Input: dimensioned drawing with shaded views. Units: mm. Origin: part minimum x, y, z. A direction names the side the tool comes from. Round coordinates to 2 decimals unless told otherwise and drop trailing zeros. Loops run counter-clockwise (first coordinate to the right, second up) from the corner with the lowest first, then second, coordinate; pieces in that order, holes last.
Item 1: Section query A-A on z = 4. Return loops of the section in (x, y).
Item 2: Ray query, L1, parallel to X at y = 0.75, z = 4; L2, parallel to Y at x = 7.25, z = 2; L3, parallel to Y at x = 2.75, z = 4.75. Return the intervals inside material, ascending.
Item 3: First-contact query: P1, Ø3, axis at x = 3.95, z = 4, coming from the -Y side; P2, Ø1, axis at x = 9, z = 5, coming from the +Y side. Flat tips, straight axial feed; report the tip coordinate or a pass-through.
Item 4: Pull-direction query (X, two-part tool) for the marked faces 1, 2, 3 and 4; classes: released by +X, released by -X, zero draft, split by the parting line, or undercut.
Item 5: Section query D-D on z = 6.75. Return loops of the section in (x, y), then the cut area to 3 significant figures.
Item 6: Section query B-B on x = 11.85. Return loops of the section in (y, z), then the cut area to 3 significant figures.
Item 7: Section query C-C on y = 0.75. Return loops of the section in (x, z).
Item 8: Access query for the marked faces 5, 6 and 7. Directions: +Z, -Z, +X, -X, +Y, -Y. A direction counts if a zero-diameter tool reaches every point of the face in a straight line with its end or side. Return the directions, or none.
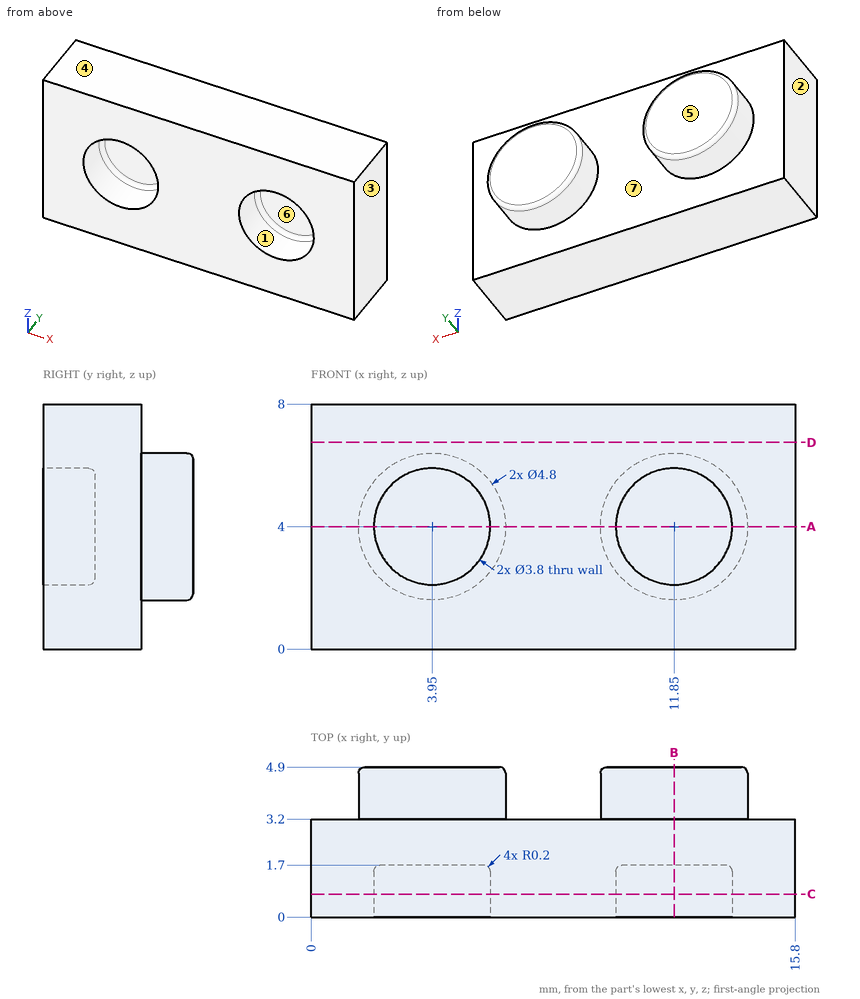
Data:
1. outline: (0, 0) - (2.05, 0) - (2.05, 1.5) arc R0.2 cw to (2.25, 1.7) - (5.65, 1.7) arc R0.2 cw to (5.85, 1.5) - (5.85, 0) - (9.95, 0) - (9.95, 1.5) arc R0.2 cw to (10.15, 1.7) - (13.55, 1.7) arc R0.2 cw to (13.75, 1.5) - (13.75, 0) - (15.8, 0) - (15.8, 3.2) - (14.25, 3.2) - (14.25, 4.7) arc R0.2 ccw to (14.05, 4.9) - (9.65, 4.9) arc R0.2 ccw to (9.45, 4.7) - (9.45, 3.2) - (6.35, 3.2) - (6.35, 4.7) arc R0.2 ccw to (6.15, 4.9) - (1.75, 4.9) arc R0.2 ccw to (1.55, 4.7) - (1.55, 3.2) - (0, 3.2) - close
2. L1: x = 0 to 2.05, 5.85 to 9.95, 13.75 to 15.8
2. L2: y = 0 to 3.2
2. L3: y = 1.7 to 4.9
3. P1: stops at y = 1.7
3. P2: stops at y = 3.2
4. face 1: undercut
4. face 2: released by -X
4. face 3: released by +X
4. face 4: zero draft
5. outline: (0, 0) - (15.8, 0) - (15.8, 3.2) - (0, 3.2) - close
5. area: 50.6 mm2
6. outline: (0, 0) - (3.2, 0) - (3.2, 1.6) - (4.7, 1.6) arc R0.2 ccw to (4.9, 1.8) - (4.9, 6.2) arc R0.2 ccw to (4.7, 6.4) - (3.2, 6.4) - (3.2, 8) - (0, 8) - (0, 5.9) - (1.5, 5.9) arc R0.2 cw to (1.7, 5.7) - (1.7, 2.3) arc R0.2 cw to (1.5, 2.1) - (0, 2.1) - close
6. area: 27.3 mm2
7. outline: (0, 0) - (15.8, 0) - (15.8, 8) - (0, 8) - close; hole circle Ø3.8 at (3.95, 4); hole circle Ø3.8 at (11.85, 4)
8. face 5: +Z, -Z, +X, -X, +Y
8. face 6: -Y
8. face 7: +Y
